Input: part model. Units: mm. Frame: model coordinates. A direction names the side the tool comes from. Coordinates: 2 decimals unless noted, no trailing zeros. Write each loop counter-clockwise with the first axis right and the second up, starting at its lowest first coordinate (ties: lowest second). Pieces come first, ordered by that corner, then holes. Notation, with made-up numbers: (35.25, 48.5) -> (48.25, 48.5) arc R13 ccw to (48.25, 55.5) -> close; hole circle Ø10 at (7, 78.5). An arc over 180 degrees is marked (long way). Use one line per item in the form item = value. Start each with the question number.
(1) Cut plane D-D on z = 10. Return the cut outline in (x, y), plus the area to 3 significant figures.
(2) First-contact query: pin 1 (4.5 mm diameter, centred on x = 316, z = 24, fed in from +Y); pin 2 (3.5 mm diameter, centred on y = 66, z = 25, fed in from -X); pin 3 (6.5 mm diameter, centred on x = 321, y = 35, fed in from +Z). Flat tips, straight axial feed; report the tip coordinate or a pass-through.
(3) Set-up query: faces 4 (the face through (322, 37, 13.5)), 5 (the face through (256, 37, 13.5)), 6 (the face through (264, 63, 20.2)). Return all of +Z, -Z, +X, -X, +Y, -Y with unobstructed straight access to the full face (end or side cutting, diameter ignored); none if empty.
(4) Cut plane C-C on y = 21. Return the cut outline in (x, z).
(5) Cut plane A-A on x = 316. Return the cut outline in (y, z).
(6) Cut plane B-B on z = 28.5. Return the cut outline in (x, y), plus the area to 3 significant figures.
(7) Pull-direction query (Y, two-part tool) for faces 1 (the face through (257.825, 38.606, 15.255)), 2 (the face through (325.185, 43.059, 15.305)), 3 (the face through (313, 14, 20.2)); classes: released by +Y, released by -Y, zero draft, split by the parting line, or undercut.
(8) Ray query, line 1 along X through (y, z) = (58.5, 10.5); line 2 along X through (y, z) = (38, 14.5); line 3 along Z through (x, y) = (314, 62). Return the intervals inside material, ascending.
```python
from build123d import *

# Parameters (mm, degrees)
SKETCH_1_W          = 57.2
SKETCH_1_H          = 57.2
EXTRUDE_1_DEPTH     = 20.2
EXTRUDE_2_DEPTH     = 11
FILLET_1_R          = 4
SKETCH_3_W          = 8.36
SKETCH_3_H          = 10.17
EXTRUDE_3_DEPTH     = 3.56
FILLET_2_R          = 2
CUT_EXTRUDE_1_REACH = 335.105
SKETCH_4_R          = 1.4


with BuildPart() as part:
    # 草图1 → 凸台-拉伸1 (new body)
    with BuildSketch(Plane.XY):
        with Locations((288.826790697, 38.544140377)):
            Rectangle(SKETCH_1_W, SKETCH_1_H)
    extrude(amount=EXTRUDE_1_DEPTH)

    # 草图2 → 凸台-拉伸2 (add)
    with BuildSketch(Plane.XY.offset(20.2)):
        Polygon((260.226790697, 58.884140377), (268.486790697, 58.884140377), (268.486790697, 67.144140377), (309.166790697, 67.144140377), (309.166790697, 58.884140377), (317.426790697, 58.884140377), (317.426790697, 18.204140377), (309.166790697, 18.204140377), (309.166790697, 9.944140377), (268.486790697, 9.944140377), (268.486790697, 18.204140377), (260.226790697, 18.204140377), align=None)
    extrude(amount=EXTRUDE_2_DEPTH)

    # 圆角1
    fillet_1_edges = [part.edges().sort_by_distance(p)[0] for p in [
        (268.486790697, 58.884140377, 25.7),
        (268.486790697, 18.204140377, 25.7),
        (309.166790697, 18.204140377, 25.7),
        (309.166790697, 58.884140377, 25.7),
    ]]
    fillet(fillet_1_edges, radius=FILLET_1_R)

    # 草图3 → 凸台-拉伸3 (add)
    with BuildSketch(Plane(origin=(0, 0, 13.5), x_dir=(-1, 0, 0), z_dir=(0, 0, -1))):
        with Locations((-256.046790697, 38.544140377)):
            Rectangle(SKETCH_3_W, SKETCH_3_H)
        with Locations((-321.606790697, 38.544140377)):
            Rectangle(SKETCH_3_W, SKETCH_3_H)
    extrude(amount=-EXTRUDE_3_DEPTH)

    # 圆角2
    fillet_2_edges = [part.edges().sort_by_distance(p)[0] for p in [
        (251.866790697, 43.629140377, 15.28),
        (251.866790697, 33.459140377, 15.28),
        (260.226790697, 33.459140377, 15.28),
        (260.226790697, 43.629140377, 15.28),
        (317.426790697, 43.629140377, 15.28),
        (317.426790697, 33.459140377, 15.28),
        (325.786790697, 33.459140377, 15.28),
        (325.786790697, 43.629140377, 15.28),
    ]]
    fillet(fillet_2_edges, radius=FILLET_2_R)

    # 草图4 → 切除-拉伸1 (cut, up to next)
    with BuildSketch(Plane(origin=(0, 0, 13.5), x_dir=(-1, 0, 0), z_dir=(0, 0, -1)), mode=Mode.PRIVATE) as cut_extrude_1_sk1:
        with Locations((-256.426790697, 38.544140377)):
            Circle(SKETCH_4_R)
    cut_extrude_1_tool1 = extrude(cut_extrude_1_sk1.sketch, amount=-CUT_EXTRUDE_1_REACH, mode=Mode.PRIVATE) & part.part
    # 草图4 → 切除-拉伸1 (cut, up to next)
    with BuildSketch(Plane(origin=(0, 0, 13.5), x_dir=(-1, 0, 0), z_dir=(0, 0, -1)), mode=Mode.PRIVATE) as cut_extrude_1_sk2:
        with Locations((-321.226790697, 38.544140377)):
            Circle(SKETCH_4_R)
    cut_extrude_1_tool2 = extrude(cut_extrude_1_sk2.sketch, amount=-CUT_EXTRUDE_1_REACH, mode=Mode.PRIVATE) & part.part
    add(cut_extrude_1_tool1.solids().sort_by_distance((256.426791, 38.54414, 13.5))[0], mode=Mode.SUBTRACT)
    add(cut_extrude_1_tool2.solids().sort_by_distance((321.226791, 38.54414, 13.5))[0], mode=Mode.SUBTRACT)


solid = part.part
```
Values:
q1.outline = (260.23, 9.94) -> (317.43, 9.94) -> (317.43, 67.14) -> (260.23, 67.14) -> close
q1.area = 3,270 mm2
q2.pin_1 = 58.88
q2.pin_2 = 268.49
q2.pin_3 = 17.06
q3.face_4 = -Z, +X, +Y, -Y
q3.face_5 = -Z, -X, +Y, -Y
q3.face_6 = +Z, -X, +Y
q4.outline = (260.23, 0) -> (317.43, 0) -> (317.43, 31.2) -> (260.23, 31.2) -> close
q5.outline = (9.94, 0) -> (67.14, 0) -> (67.14, 20.2) -> (58.88, 20.2) -> (58.88, 31.2) -> (18.2, 31.2) -> (18.2, 20.2) -> (9.94, 20.2) -> close
q6.outline = (260.23, 18.2) -> (264.49, 18.2) arc R4 cw to (268.49, 14.2) -> (268.49, 9.94) -> (309.17, 9.94) -> (309.17, 14.2) arc R4 cw to (313.17, 18.2) -> (317.43, 18.2) -> (317.43, 58.88) -> (313.17, 58.88) arc R4 cw to (309.17, 62.88) -> (309.17, 67.14) -> (268.49, 67.14) -> (268.49, 62.88) arc R4 cw to (264.49, 58.88) -> (260.23, 58.88) -> close
q6.area = 3,010 mm2
q7.face_1 = undercut
q7.face_2 = released by +Y
q7.face_3 = zero draft
q8.line_1 = 260.23 to 317.43
q8.line_2 = 251.87 to 255.14, 257.72 to 319.94, 322.52 to 325.79
q8.line_3 = 0 to 20.2
